Input: part model. Units: mm. Frame: model coordinates. Round coordinates to 2 decimals unless told otherwise and drop trailing zeros. Write each loop counter-clockwise with the first axis right and the second up, starting at its lowest first coordinate (ties: lowest second). Pieces come first, ordered by that corner, then holes. Notation, with made-up numbers: (36, -19.5) - (49, -19.5) arc R20 cw to (49, 17.5) - close; hole circle Ø9 at (67, 58.5). An arc over 180 degrees is marked (long way). One line per item, written item: value. Start each with the question number.
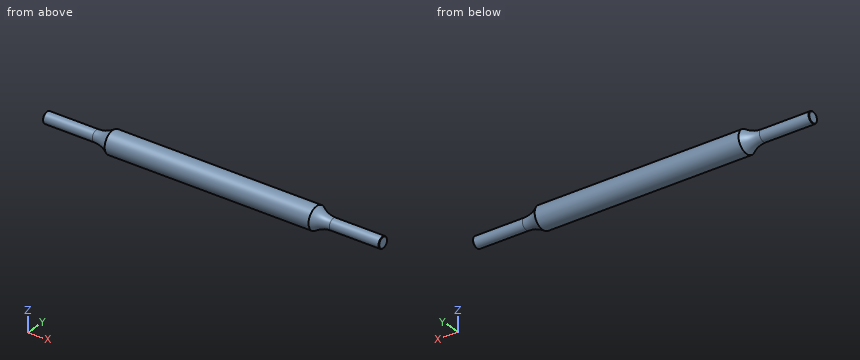
```python
from build123d import *

# Parameters (mm, degrees)
CHAMFER1_SIZE = 0.075


with BuildPart() as part:
    # Sketch1 → Revolve1 (revolve)
    with BuildSketch(Plane.XY, mode=Mode.PRIVATE) as revolve1_sk:
        with BuildLine():
            Line((-30.49, 0), (30.49, 0))
            Line((30.49, 0), (30.49, 1))
            Line((30.49, 1), (21.49, 1))
            ThreePointArc((21.49, 1), (19.90886117, 1.25658351), (18.49, 2))
            Line((18.49, 2), (-18.49, 2))
            ThreePointArc((-18.49, 2), (-19.90886117, 1.25658351), (-21.49, 1))
            Line((-21.49, 1), (-30.49, 1))
            Line((-30.49, 1), (-30.49, 0))
        make_face()
    revolve(revolve1_sk.sketch.rotate(Axis((-30.49, 0, 0), (1, 0, 0)), 90), axis=Axis((-30.49, 0, 0), (1, 0, 0)))

    # Chamfer1
    chamfer1_edges = [part.edges().sort_by_distance(p)[0] for p in [
        (-30.49, 0, -1),
        (30.49, 0, -1),
    ]]
    chamfer(chamfer1_edges, length=CHAMFER1_SIZE)


solid = part.part
```
Q1. Contact query for flat-ended pins moving along their axis: pin 1 Ø1.5 at (x, z) = (-22.5, -0.5) entering from +Y; pin 2 Ø2 at (x, y) = (22, -0.5) entering from -Z. Output: stop coordinate, or through.
Q2. Cut plane C-C, the plane x = -25.5. Output: boundary loops of the cut face in (y, z).
Q3. Cut plane D-D, the plane x = -14. Output: boundary loops of the cut face in (y, z), and give its area (3 significant figures).
Q4. Cut plane A-A, the plane z = 0. Output: boundary loops of the cut face in (x, y) (3 decimals).
Q5. Material intervals for probe 1 along Z at (x, y) = (-11, -0.2); probe 2 along Y at (x, z) = (14.5, -0.1); probe 3 along Y at (x, z) = (4, -0.7), sorted ascending. Write a range as from..to.
A:
1. pin 1: stops at y = 1
1. pin 2: stops at z = -1.01
2. outline: circle Ø2 at (0, 0)
3. outline: circle Ø4 at (0, 0)
3. area: 12.6 mm²
4. outline: (-30.49, -0.925) - (-30.415, -1) - (-21.49, -1) arc R5 cw to (-18.49, -2) - (18.49, -2) arc R5 cw to (21.49, -1) - (30.415, -1) - (30.49, -0.925) - (30.49, 0.925) - (30.415, 1) - (21.49, 1) arc R5 cw to (18.49, 2) - (-18.49, 2) arc R5 cw to (-21.49, 1) - (-30.415, 1) - (-30.49, 0.925) - close
5. probe 1: z = -1.99..1.99
5. probe 2: y = -2..2
5. probe 3: y = -1.87..1.87
